Read the model definition and answer for the solid it produces. Units are mm, in the model's axes. Face numbers are marked on the shaded views. A direction names the side the tool comes from. Give positions to 0.01 mm unless a question says otherwise; leave off trailing zeros. Loops run counter-clockwise (first coordinate to the right, second up) from the corner with the lowest first, then second, coordinate; pieces in that order, holes last. Notation, with made-up numbers: (9.25, -27.5) - (63.25, -27.5) arc R26 cw to (63.25, 2.5) - close; hole circle Ø6 at (-5, 40). An arc over 180 degrees is marked (long way). Write each question's results on one line, items separated by ' | '. Start each with the question number.
Q1. Find the intervals of material crossed by line 1 (Z direction, x = 1.65, y = 4); line 2 (Y direction, x = 2.15, z = 7.5); line 3 (Y direction, x = 2.55, z = -7.5), in increasing order. Write a range as from..to.
Q2. The part is cut by section B-B, the plane y = 30. Write down the section's boundary in (x, z), plus the area to 3 significant figures.
Q3. The part is cut by section A-A, the plane z = 7.5. Write down the section's boundary in (x, y), plus the area to 3 significant figures.
Q4. The part is cut by section D-D, the plane x = 26. Write down the section's boundary in (y, z), plus the area to 3 significant figures.
Q5. The part is cut by section C-C, the plane y = 12.5. Write down the section's boundary in (x, z).
Q6. Given pin 1 (8 mm diameter, centred on x = -4.5, y = 26, fed in from +Z); pin 2 (7 mm diameter, centred on y = 4, z = -7.5, fed in from +X); pin 3 (1 mm diameter, centred on x = -2, z = 0, fed in from -Y); pin 4 (2.5 mm diameter, centred on x = 2, z = 5.5, fed in from +Y), each flat-ended and moving along its own axis, determine where each tip first touches the part or whether it passes through.
Q7. For the marked faces 1 and 2, determine the directions among +Z, -Z, +X, -X, +Y, -Y from which every point of the face is accessible in a straight line to the end or side of a thin tool.
```python
from build123d import *

# Parameters (mm, degrees)
EXTRUDE_1_DEPTH          = 1.6
EXTRUDE_1_DEPTH_BACK     = 1.6
EXTRUDE_2_DEPTH          = 11.5
EXTRUDE_2_DEPTH_BACK     = 11.5
SKETCH_2_W               = 3.2
SKETCH_2_H               = 34
CUT_EXTRUDE_1_DEPTH      = 87.501676284
CUT_EXTRUDE_1_DEPTH_BACK = 87.501676284
SKETCH_3_R               = 2.25


with BuildPart() as part:
    # ｽｹｯﾁ1 → ﾎﾞｽ - 押し出し1 (new, two sides: drawn at the far end of the back side and taken through both)
    with BuildSketch(Plane.XY.offset(-EXTRUDE_1_DEPTH_BACK)):
        with BuildLine():
            Line((3.2, 0), (34.7, 0))
            ThreePointArc((34.7, 0), (36.821320344, 0.878679656), (37.7, 3))
            Line((37.7, 3), (37.7, 57))
            Line((37.7, 57), (17.7, 77))
            Line((17.7, 77), (-6.8, 77))
            ThreePointArc((-6.8, 77), (-8.921320344, 76.121320344), (-9.8, 74))
            Line((-9.8, 74), (-9.8, 50))
            ThreePointArc((-9.8, 50), (-8.921320344, 47.878679656), (-6.8, 47))
            Line((-6.8, 47), (3.2, 47))
            Line((3.2, 47), (3.2, 0))
        make_face()
    extrude(amount=EXTRUDE_1_DEPTH + EXTRUDE_1_DEPTH_BACK)

    # ｽｹｯﾁ2 → ﾎﾞｽ - 押し出し2 (add, two sides: drawn at the far end of the back side and taken through both)
    with BuildSketch(Plane.XY.offset(-EXTRUDE_2_DEPTH_BACK)):
        with Locations((1.6, 17)):
            Rectangle(SKETCH_2_W, SKETCH_2_H)
    extrude(amount=EXTRUDE_2_DEPTH + EXTRUDE_2_DEPTH_BACK)

    # ｽｹｯﾁ3 → ｶｯﾄ - 押し出し1 (cut, two sides: drawn at the far end of the back side and taken through both)
    with BuildSketch(Plane(origin=(0, 0, 0), x_dir=(0, 0, -1), z_dir=(1, 0, 0)).offset(-CUT_EXTRUDE_1_DEPTH_BACK)):
        with Locations((-7.5, 30)):
            Circle(SKETCH_3_R)
        with Locations((7.5, 4)):
            Circle(SKETCH_3_R)
    extrude(amount=CUT_EXTRUDE_1_DEPTH + CUT_EXTRUDE_1_DEPTH_BACK, mode=Mode.SUBTRACT)


solid = part.part
```
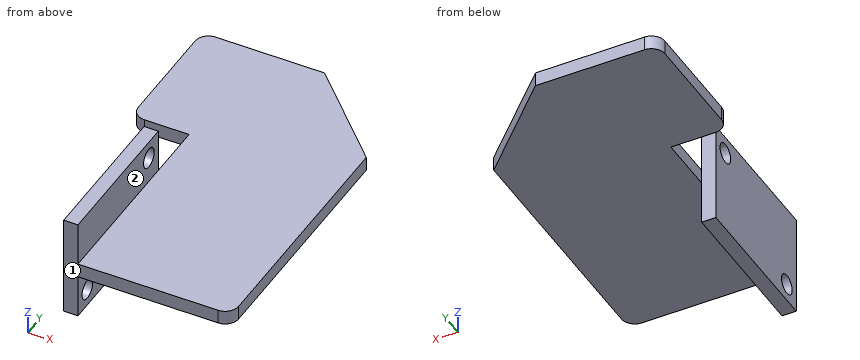
Check sheet entries:
1) line 1: z = -11.5..-9.75, -5.25..11.5 | line 2: y = 0..27.75, 32.25..34 | line 3: y = 0..1.75, 6.25..34
2) outline: (0, -11.5) - (3.2, -11.5) - (3.2, -1.6) - (37.7, -1.6) - (37.7, 1.6) - (3.2, 1.6) - (3.2, 5.25) - (0, 5.25) - close; (0, 9.75) - (3.2, 9.75) - (3.2, 11.5) - (0, 11.5) - close | area: 170 mm^2
3) outline: (0, 0) - (3.2, 0) - (3.2, 27.75) - (0, 27.75) - close; (0, 32.25) - (3.2, 32.25) - (3.2, 34) - (0, 34) - close | area: 94.4 mm^2
4) outline: (0, -1.6) - (68.7, -1.6) - (68.7, 1.6) - (0, 1.6) - close | area: 220 mm^2
5) outline: (0, -11.5) - (3.2, -11.5) - (3.2, -1.6) - (37.7, -1.6) - (37.7, 1.6) - (3.2, 1.6) - (3.2, 11.5) - (0, 11.5) - close
6) pin 1: passes through | pin 2: stops at x = 3.2 | pin 3: stops at y = 47 | pin 4: stops at y = 34
7) face 1: +Z, -Z, +X, -X, -Y | face 2: +Z, +X, +Y, -Y
